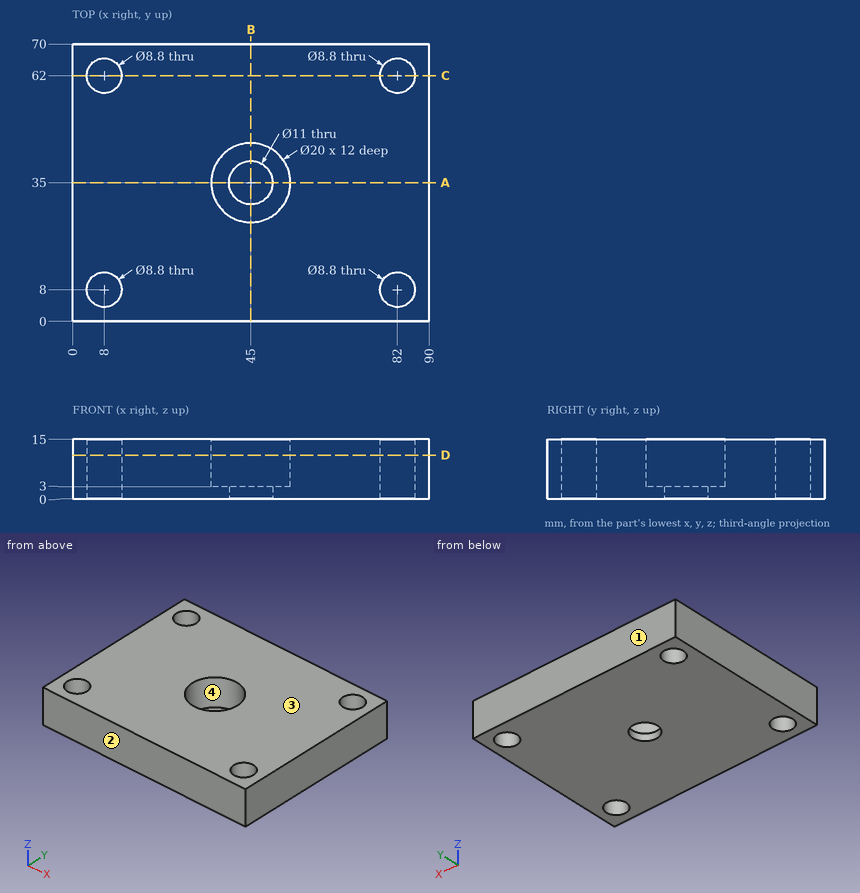
Verification items for this drawing (mm, ordinates from the low corner). Give positions to 0.01 mm unless a question says otherwise; leave off trailing zeros. Loops run counter-clockwise (first coordinate to the right, second up) from the corner with the lowest first, then second, coordinate; pieces in that order, holes last. Notation, with made-up numbers: M 35,25 L 72,25 A11 ccw 72,32 Z; hole C 52,0.25 d7. An arc over 180 degrees is marked long. Answer in a Markdown table with one row per item.
1) Mould release check, pull along Y, two halves, no side actions. Record for the marked faces 1, 2, 3 and 4: released by +Y, released by -Y, zero draft, split by the parting line, or undercut.
Solutions:
| item | result |
|---|---|
| face 1 | released by +Y |
| face 2 | released by -Y |
| face 3 | zero draft |
| face 4 | undercut |
2) Cross-section at B-B (x = 45). Enter the section's corners in (y, z), plus the area to 3 significant figures.
Solutions:
| item | result |
|---|---|
| outline | M 0,0 L 29.5,0 L 29.5,3 L 25,3 L 25,15 L 0,15 Z; M 40.5,0 L 70,0 L 70,15 L 45,15 L 45,3 L 40.5,3 Z |
| area | 777 mm^2 |
3) Cross-section at D-D (z = 11). Enter the section's corners in (x, y).
Solutions:
| item | result |
|---|---|
| outline | M 0,0 L 90,0 L 90,70 L 0,70 Z; hole C 8,8 d8.8; hole C 8,62 d8.8; hole C 45,35 d20; hole C 82,8 d8.8; hole C 82,62 d8.8 |
4) Thickness scan on line 1 (Y direction, x = 82, z = 6.75); line 2 (Y direction, x = 45, z = 7); line 3 (X direction, y = 66, z = 3). Record the ranges inside material, lowest first.
Solutions:
| item | result |
|---|---|
| line 1 | y = 0 to 3.6, 12.4 to 57.6, 66.4 to 70 |
| line 2 | y = 0 to 25, 45 to 70 |
| line 3 | x = 0 to 6.17, 9.83 to 80.17, 83.83 to 90 |
5) Cross-section at A-A (y = 35). Enter the section's corners in (x, z), plus the area to 3 significant figures.
Solutions:
| item | result |
|---|---|
| outline | M 0,0 L 39.5,0 L 39.5,3 L 35,3 L 35,15 L 0,15 Z; M 50.5,0 L 90,0 L 90,15 L 55,15 L 55,3 L 50.5,3 Z |
| area | 1,080 mm^2 |
6) Cross-section at C-C (y = 62). Enter the section's corners in (x, z).
Solutions:
| item | result |
|---|---|
| outline | M 0,0 L 3.6,0 L 3.6,15 L 0,15 Z; M 12.4,0 L 77.6,0 L 77.6,15 L 12.4,15 Z; M 86.4,0 L 90,0 L 90,15 L 86.4,15 Z |
7) Depth check by flat-ended pin: pin 1 (6 mm diameter, centred on x = 41, y = 31.5, fed in from +Z). Enter the tip coordinate at first touch or a pass-through.
Solutions:
| item | result |
|---|---|
| pin 1 | stops at z = 3 |
